Source: CAD feature listing. Evaluate the final solid. Frame: model axes, mm. Face numbers are marked on the shaded views. A direction names the side the tool comes from. Round coordinates to 2 decimals unless told otherwise and drop trailing zeros. Order: outer loops, then holes, each group sorted by start corner. A loop starts at its lowest first (then second) coordinate and runs counter-clockwise, first axis right, second up.
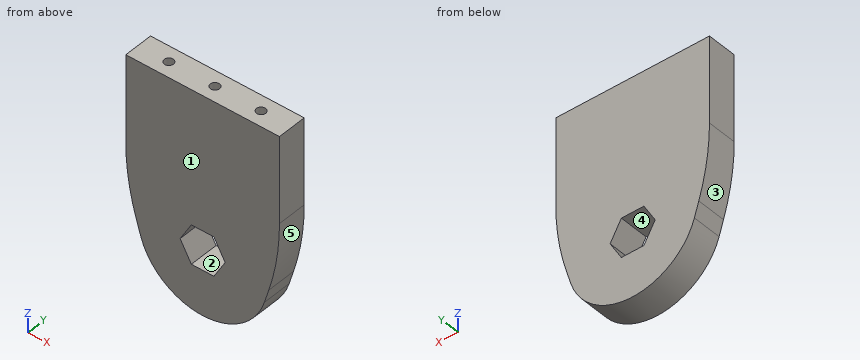
```python
from build123d import *

# Parameters (mm, degrees)
CROQUIS1_R              = 21
CROQUIS1_W              = 50
CROQUIS1_H              = 40
SALIENTE_EXTRUIR1_DEPTH = 9.6
CROQUIS2_R              = 16
CORTAR_EXTRUIR1_DEPTH   = 58.603472118
REDONDEO1_R             = 80
CROQUIS3_R              = 1.5
CORTAR_EXTRUIR2_DEPTH   = 15
MATRIZL1_COUNT          = 2
MATRIZL1_PITCH          = 15
MATRIZL1_COL_COUNT      = 2
MATRIZL1_COL_PITCH      = 15
SKETCH1_R               = 16
BOSS_EXTRUDE1_DEPTH     = 9.6
SKETCH3_R               = 10
BOSS_EXTRUDE2_DEPTH     = 9.6
CUT_EXTRUDE2_DEPTH      = 10


with BuildPart() as part:
    # Croquis1 → Saliente-Extruir1 (new body)
    with BuildSketch(Plane(origin=(0, 0, 0), x_dir=(1, 0, 0), z_dir=(0, 1, 0))):
        with Locations((0, 30)):
            Circle(CROQUIS1_R)
        Rectangle(CROQUIS1_W, CROQUIS1_H)
        with BuildLine():
            ThreePointArc((20.088252282, 36.120630706), (0, 51), (-20.088252282, 36.120630706))
            ThreePointArc((-20.088252282, 36.120630706), (-20.89449325, 27.897584284), (-18.466185313, 20))
            Line((-18.466185313, 20), (18.466185313, 20))
            ThreePointArc((18.466185313, 20), (20.356692899, 24.841991255), (21, 30))
            ThreePointArc((21, 30), (20.770812429, 33.09408323), (20.088252282, 36.120630706))
        make_face()
        with BuildLine():
            Line((18.466185313, 20), (-18.466185313, 20))
            ThreePointArc((-18.466185313, 20), (0, 9), (18.466185313, 20))
        make_face()
        with BuildLine():
            Line((25, 20), (20.088252282, 36.120630706))
            ThreePointArc((20.088252282, 36.120630706), (20.770812429, 33.09408323), (21, 30))
            ThreePointArc((21, 30), (20.356692899, 24.841991255), (18.466185313, 20))
            Line((18.466185313, 20), (25, 20))
        make_face()
        with BuildLine():
            Line((-20.088252282, 36.120630706), (-25, 20))
            Line((-25, 20), (-18.466185313, 20))
            ThreePointArc((-18.466185313, 20), (-20.89449325, 27.897584284), (-20.088252282, 36.120630706))
        make_face()
    extrude(amount=SALIENTE_EXTRUIR1_DEPTH)

    # Croquis2 → Cortar-Extruir1 (cut, through all)
    with BuildSketch(Plane(origin=(0, 9.6, 0), x_dir=(1, 0, 0), z_dir=(0, 1, 0))):
        with Locations(Location((0, 30, 0), (0, 0, 270))):
            Circle(CROQUIS2_R)
    extrude(amount=-CORTAR_EXTRUIR1_DEPTH, mode=Mode.SUBTRACT)

    # Redondeo1
    redondeo1_edges = [part.edges().sort_by_distance(p)[0] for p in [
        (25, 4.8, -20),
        (-25, 4.8, -20),
    ]]
    fillet(redondeo1_edges, radius=REDONDEO1_R)

    # Croquis3 → Cortar-Extruir2 (cut)
    with BuildSketch(Plane.XY.offset(20)):
        with Locations((0, 4.8)):
            Circle(CROQUIS3_R)
    cortar_extruir2 = extrude(amount=-CORTAR_EXTRUIR2_DEPTH, mode=Mode.SUBTRACT)

    # MatrizL1: Cortar-Extruir2 ×2
    with Locations(*[(i * MATRIZL1_PITCH, 0, 0) for i in range(1, MATRIZL1_COUNT)]):
        add(cortar_extruir2, mode=Mode.SUBTRACT)

    # MatrizL1 col: Cortar-Extruir2 ×2
    with Locations(*[(-i * MATRIZL1_COL_PITCH, 0, 0) for i in range(1, MATRIZL1_COL_COUNT)]):
        add(cortar_extruir2, mode=Mode.SUBTRACT)

    # Sketch1 → Boss-Extrude1 (add)
    with BuildSketch(Plane(origin=(0, 9.6, 0), x_dir=(1, 0, 0), z_dir=(0, 1, 0))):
        with Locations((0, 30)):
            Circle(SKETCH1_R)
        with BuildLine():
            Line((-2.5, 36.538348415), (-2.5, 39.5))
            Line((-2.5, 39.5), (2.5, 39.5))
            Line((2.5, 39.5), (2.5, 36.538348415))
            ThreePointArc((2.5, 36.538348415), (5.766281297, 33.968626967), (7, 30))
            ThreePointArc((7, 30), (-3.968626967, 24.233718703), (-2.5, 36.538348415))
        make_face(mode=Mode.SUBTRACT)
    extrude(amount=-BOSS_EXTRUDE1_DEPTH)

    # Sketch3 → Boss-Extrude2 (add)
    with BuildSketch(Plane(origin=(0, 9.6, 0), x_dir=(1, 0, 0), z_dir=(0, 1, 0))):
        with Locations((0, 30)):
            Circle(SKETCH3_R)
    extrude(amount=-BOSS_EXTRUDE2_DEPTH)

    # Sketch2 → Cut-Extrude2 (cut)
    with BuildSketch(Plane(origin=(0, 9.6, 0), x_dir=(1, 0, 0), z_dir=(0, 1, 0))):
        Polygon((3.666174209, 36.35), (-3.666174209, 36.35), (-7.332348419, 30), (-3.666174209, 23.65), (3.666174209, 23.65), (7.332348419, 30), align=None)
    extrude(amount=-CUT_EXTRUDE2_DEPTH, mode=Mode.SUBTRACT)


solid = part.part
```
1. Section A-A on x = 0. Return loops of the section in (y, z), plus the area to 3 significant figures.
2. Section D-D on x = -14.5. Return loops of the section in (y, z).
3. Access query for the marked faces 4 and 5. Directions: +Z, -Z, +X, -X, +Y, -Y. A direction counts if a zero-diameter tool reaches every point of the face in a straight line with its end or side. Return the directions, or none.
4. Pull-direction query (X, two-part tool) for the marked faces 1, 2 and 3; classes: released by +X, released by -X, zero draft, split by the parting line, or undercut.
5. Section B-B on y = 7.75. Return loops of the section in (x, z).
6. First-contact query: pin 1 (1 mm diameter, centred on y = 5, z = -24, fed in from -X); pin 2 (8 mm diameter, centred on x = 18.5, z = -2.5, fed in from -Y); pin 3 (5 mm diameter, centred on x = 6.5, y = 7.5, fed in from -Z); pin 4 (1.5 mm diameter, centred on x = -15, y = 5.5, fed in from +Z). Flat tips, straight axial feed; report the tip coordinate or a pass-through.
7. Section C-C on z = -29. Return loops of the section in (x, y) (3 decimals).
8. Line query: line 1 along Y through (x, z) = (-15, 12); line 2 along X through (y, z) = (5.25, 14); line 3 along Z through (x, y) = (-2.5, 2). Output: solid intervals per line, ascending.
Result:
1. outline: (0, -51) - (9.6, -51) - (9.6, -36.35) - (0, -36.35) - close; (0, -23.65) - (9.6, -23.65) - (9.6, 20) - (6.3, 20) - (6.3, 5) - (3.3, 5) - (3.3, 20) - (0, 20) - close
1. area: 515 mm2
2. outline: (0, -45.19) - (9.6, -45.19) - (9.6, 20) - (6.21, 20) - (6.21, 5) - (3.39, 5) - (3.39, 20) - (0, 20) - close
3. face 4: +Y, -Y
3. face 5: -Z, +X, +Y, -Y
4. face 1: zero draft
4. face 2: undercut
4. face 3: released by -X
5. outline: (-25, -8.08) arc R80 ccw to (-21.53, -31.4) - (-20.09, -36.12) arc R21 ccw to (20.09, -36.12) - (21.53, -31.4) arc R80 ccw to (25, -8.08) - (25, 20) - (-25, 20) - close; hole (-7.33, -30) - (-3.67, -36.35) - (3.67, -36.35) - (7.33, -30) - (3.67, -23.65) - (-3.67, -23.65) - close
6. pin 1: stops at x = -23.5
6. pin 2: stops at y = 0
6. pin 3: stops at z = -50.62
6. pin 4: stops at z = 5
7. outline: (-22.217, 0) - (-6.755, 0) - (-6.755, 9.6) - (-22.217, 9.6) - close; (6.755, 0) - (22.217, 0) - (22.217, 9.6) - (6.755, 9.6) - close
8. line 1: y = 0 to 3.3, 6.3 to 9.6
8. line 2: x = -25 to -16.43, -13.57 to -1.43, 1.43 to 13.57, 16.43 to 25
8. line 3: z = -50.85 to -36.35, -23.65 to 20
